For this review, take the finished solid that the model builds, in its own axes (mm). Face numbers are marked on the shaded views. Coordinates: 2 decimals unless noted, no trailing zeros. Loops run counter-clockwise (first coordinate to the right, second up) from the corner with the lowest first, then second, coordinate; pieces in that order, holes last. Notation, with made-up numbers: M 49,62 L 108,62 A23 cw 108,99 Z; hole C -40,29.5 d1. An arc over 180 degrees is marked long. Put each result on its own line as item: value.
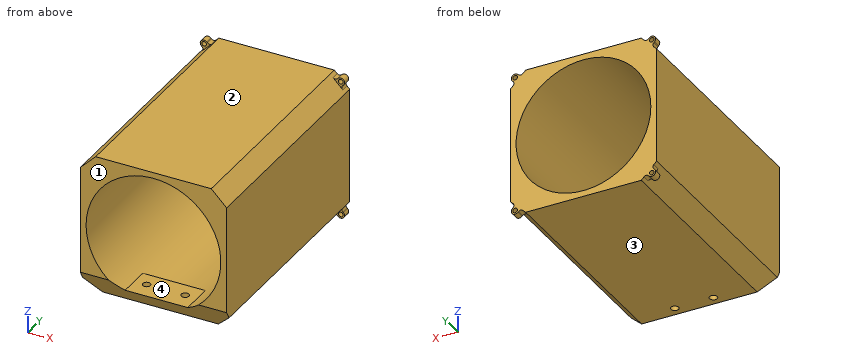
Autodesk Inventor part; units mm, degrees
ref_plane "YZ Plane" through (0, 0, 0) normal (1, 0, 0) x (0, 1, 0)
ref_plane "XZ Plane" through (0, 0, 0) normal (0, 1, 0) x (-1, 0, 0)
ref_plane "XY Plane" through (0, 0, 0) normal (0, 0, 1) x (1, 0, 0)
sketch "Sketch1" plane through (0, 0, 0) normal (0, 1, 0) x (-1, 0, 0)
  circle A0 centre (0, 0) radius 43.732
  line L0 (-47.5, -47.5) -> (47.5, -47.5)
  line L1 (47.5, -47.5) -> (47.5, 47.5)
  line L2 (47.5, 47.5) -> (-47.5, 47.5)
  line L3 (-47.5, 47.5) -> (-47.5, -47.5)
  line L4 (-47.5, -47.5) -> (47.5, 47.5) construction
  line L5 (47.5, -47.5) -> (-47.5, 47.5) construction
  dimension "d0" = 87.464
  dimension "d4" = 95
  dimension "d5" = 95
extrude "Extrusion1" add sketch "Sketch1" along normal blind 149
chamfer "Chamfer1" distance 10 angle 45 4 edges at (47.5, 74.5, -47.5) (47.5, 74.5, 47.5) (-47.5, 74.5, 47.5) (-47.5, 74.5, -47.5)
sketch "Sketch2" plane through (0, 149, 0) normal (0, 1, 0) x (1, 0, 0)
  line L0 (-47.5, 37.5) -> (-37.5, 47.5)
  line L1 (-47.5, 37.5) -> (-47.5, -37.5)
  line L2 (-37.5, -47.5) -> (-47.5, -37.5)
  line L3 (-37.5, -47.5) -> (37.5, -47.5)
  line L4 (47.5, -37.5) -> (37.5, -47.5)
  line L5 (47.5, -37.5) -> (47.5, 37.5)
  line L6 (37.5, 47.5) -> (47.5, 37.5)
  line L7 (37.5, 47.5) -> (-37.5, 47.5)
  circle A0 centre (0, 0) radius 43.732
  line L8 (-42.5, 42.5) -> (-44.3434, 44.3434)
  circle A1 centre (-44.3434, 44.3434) radius 1.5
  circle A2 centre (-44.3434, 44.3434) radius 2.5
  line L9 (-42.5757, 46.1112) -> (-40.7322, 44.2678)
  line L10 (-46.1112, 42.5757) -> (-44.2678, 40.7322)
  line L11 (0, 47.5) -> (0, 44.5)
  line L12 (-47.5, 0) -> (-44.5, 0)
  circle A3 centre (44.3434, 44.3434) radius 1.5
  circle A4 centre (44.3434, 44.3434) radius 2.5
  line L13 (42.5757, 46.1112) -> (40.7322, 44.2678)
  line L14 (46.1112, 42.5757) -> (44.2678, 40.7322)
  circle A5 centre (-44.3434, -44.3434) radius 1.5
  circle A6 centre (-44.3434, -44.3434) radius 2.5
  line L15 (-42.5757, -46.1112) -> (-40.7322, -44.2678)
  line L16 (-46.1112, -42.5757) -> (-44.2678, -40.7322)
  circle A7 centre (44.3434, -44.3434) radius 2.5
  circle A8 centre (44.3434, -44.3434) radius 1.5
  line L17 (42.5757, -46.1112) -> (40.7322, -44.2678)
  line L18 (46.1112, -42.5757) -> (44.2678, -40.7322)
  dimension "d9" = 2.607
  dimension "d10" = 3
  dimension "d11" = 1
  dimension "d12" = 3
  dimension "d13" = 3
extrude "Extrusion2" add sketch "Sketch2" against normal blind 5 contours L10 A2 L8 L0 | L8 A2 L9 L0 | A2 | L2 L15 A6 L16 | A6 | L13 A4 L14 L6 | L4 L18 A7 L17 | A4 | A7
fillet "Fillet1" radius 2 8 edges at (44.2678, 146.5, -40.7322) (40.7322, 146.5, -44.2678) (44.2678, 146.5, 40.7322) (40.7322, 146.5, 44.2678) (-40.7322, 146.5, 44.2678) (-44.2678, 146.5, 40.7322) (-44.2678, 146.5, -40.7322) (-40.7322, 146.5, -44.2678)
sketch "Sketch5" plane through (0, 0, 0) normal (0, -1, 0) x (1, 0, 0)
  line L0 (-37.5, -47.5) -> (-47.5, -37.5)
  line L1 (37.5, -47.5) -> (-37.5, -47.5)
  line L2 (47.5, -37.5) -> (37.5, -47.5)
  line L3 (47.5, 37.5) -> (47.5, -37.5)
  line L4 (37.5, 47.5) -> (47.5, 37.5)
  line L5 (-37.5, 47.5) -> (37.5, 47.5)
  line L6 (-47.5, 37.5) -> (-37.5, 47.5)
  line L7 (-47.5, -37.5) -> (-47.5, 37.5)
  circle A0 centre (0, 0) radius 43.732
  circle A1 centre (0, 0) radius 43.732
  line L8 (0, -43.732) -> (0, -38.732)
  line L9 (-20.3057, -38.732) -> (20.3057, -38.732)
  dimension "d30" = 5
extrude "Extrusion4" add sketch "Sketch5" against normal blind 25 contours L9 L8 A0 | A0 L8 L9
sketch "Sketch6" plane through (37.5, 0, -47.5) normal (0, 0, -1) x (-1, 0, 0)
  line L0 (0, 0) -> (75, 0)
  line L1 (37.5, 0) -> (37.5, 15)
  line L2 (37.5, 15) -> (25, 15)
  circle A0 centre (25, 15) radius 2.5
  circle A1 centre (50, 15) radius 2.5
  dimension "d31" = 15
  dimension "d32" = 12.5
  dimension "d33" = 5
extrude "Extrusion5" cut sketch "Sketch6" against normal blind 30
sketch "Sketch7" plane through (-47.5, 0, -37.5) normal (-1, 0, 0) x (0, 0, 1)
  line L0 (0, 0) -> (0, 149)
  line L1 (0, 0) -> (75, 0)
  line L2 (75, 149) -> (75, 0)
  line L3 (0, 149) -> (75, 149)
  line L4 (-8.182, 149) -> (-8.182, 144)
  line L5 (-8.182, 149) -> (-10, 149)
  line L6 (-10, 149) -> (-10, 0)
  line L7 (-10, 0) -> (0, 0)
  line L8 (0, 0) -> (0, 149)
  line L9 (0, 149) -> (-1.818, 149)
  line L10 (-1.818, 144) -> (-1.818, 149)
  line L11 (-1.818, 144) -> (-8.182, 144)
  line L12 (0, 149) -> (0, 0)
  line L13 (0, 0) -> (14.1421, 0) construction
  line L14 (-10, 0) -> (5, 0)
  line L15 (5, 0) -> (-10, 8.6603)
  point P0 (37.5, 0)
  dimension "d39" = 15
  dimension "d40" = 30
extrude "Extrusion7" cut sketch "Sketch7" against normal through all contours L7 L6 L15 L0 | L0 L15 L1
sketch "Sketch8" plane through (-37.5, 0, 47.5) normal (0, 0, 1) x (1, 0, 0)
  line L0 (75, 0) -> (0, 0) construction
  line L1 (0, 0) -> (0, 75) construction
  line L2 (0, 75) -> (75, 75) construction
  line L3 (75, 75) -> (75, 0) construction
  point P0 (37.5, 0)
  dimension "d0" = 87.464
  dimension "d4" = 95
  dimension "d5" = 95
properties part number "Tank"
(1) Add section A-A (y = 15). Write out the cut boundary in (x, z).
Determined:
outline: M -47.5,-37.5 L -37.5,-47.5 L -15,-47.5 L -15,-38.73 L -20.31,-38.73 A43.73 cw long 20.31,-38.73 L 15,-38.73 L 15,-47.5 L 37.5,-47.5 L 47.5,-37.5 L 47.5,37.5 L 37.5,47.5 L -37.5,47.5 L -47.5,37.5 Z; M -10,-47.5 L 10,-47.5 L 10,-38.73 L -10,-38.73 Z
(2) Add section B-B (x = 0). Write out the cut boundary in (y, z).
Determined:
outline: M 0,43.73 L 149,43.73 L 149,47.5 L 0,47.5 Z; M 3.6,-38.73 L 8.66,-47.5 L 149,-47.5 L 149,-43.73 L 25,-43.73 L 25,-38.73 Z
(3) For pin 1 (8.5 mm diameter, centred on x = -43.5, z = -42.5, fed in from -Y); pin 2 (2.5 mm diameter, centred on x = -44.34, z = -44.34, fed in from +Y); pin 3 (5 mm diameter, centred on x = -44.34, z = 44.34, fed in from +Y); pin 4 (6 mm diameter, centred on x = 42.5, z = -41.5, fed in from -Y), all flat-tipped, find the tip position at first contact; note any pin that passes through.
Determined:
pin 1: stops at y = 3.32
pin 2: passes through
pin 3: stops at y = 149
pin 4: stops at y = 3.46
(4) Add section C-C (z = 0). Write out the cut boundary in (x, y), plus the area to 3 significant figures.
Determined:
outline: M -47.5,0 L -43.73,0 L -43.73,149 L -47.5,149 Z; M 43.73,0 L 47.5,0 L 47.5,149 L 43.73,149 Z
area: 1,120 mm^2
(5) Wall thickness on line 1 along Z through (x, y) = (-0.5, 126); line 2 along X through (y, z) = (28, 22.5): over which ranges is each line inside the solid? List them lowest first. Write a range as [from, to].
Determined:
line 1: z = [-47.5, -43.73], [43.73, 47.5]
line 2: x = [-47.5, -37.5], [37.5, 47.5]
(6) Draft analysis for pull direction Z (two halves, no side actions). For the marked faces 1, 2, 3 and 4, state which applies: +Z half, -Z half, draft (parallel to the pull), parting line (faces both ways), or undercut.
Determined:
face 1: draft
face 2: +Z half
face 3: -Z half
face 4: undercut
(7) Add section D-D (y = 124). Write out the cut boundary in (x, z), plus the area to 3 significant figures.
Determined:
outline: M -47.5,-37.5 L -37.5,-47.5 L 37.5,-47.5 L 47.5,-37.5 L 47.5,37.5 L 37.5,47.5 L -37.5,47.5 L -47.5,37.5 Z; hole C 0,0 d87.46
area: 2,820 mm^2
